Part model, mm, in its own coordinate system. Face numbers are marked on the shaded views. A direction names the side the tool comes from. Coordinates: 2 decimals unless noted, no trailing zeros. Loops run counter-clockwise (first coordinate to the right, second up) from the corner with the lowest first, then second, coordinate; pieces in that order, holes last. Notation, with made-up numbers: (60, 50) - (86, 50) arc R17 ccw to (86, 82) - close; hole circle Ø10 at (64, 21.5). An arc over 180 degrees is marked (long way). Use a Markdown table: item, result. Add a question column.
1. 3-axis set-ups, long thin cutter, end or side, ignore diameter. For the marked faces 5 and 6: which of +Z, -Z, +X, -X, +Y, -Y reach the whole face in a straight line?
2. Band-saw the part on D-D, the plane z = 20.25. Give the cut face in (x, y), plus the area to 3 significant figures.
3. Drop flat-ended pins along their axis: pin 1 (3 mm diameter, centred on x = 0, y = 0, fed in from -Z); pin 2 (2 mm diameter, centred on x = -13.5, z = 23.5, fed in from +Y); pin 3 (6 mm diameter, centred on x = 11.5, y = 11, fed in from -Z); pin 4 (5 mm diameter, centred on x = 8, y = -8.5, fed in from +Z). Give the stop position or say it passes through.
4. Pull direction Y, two halves, no side cores. Call the marked faces 1, 2, 3 and 4: pulls with the +Y half, pulls with the -Y half, needs draft (parallel to the pull), parting line crosses it, or undercut.
5. Wall check: probe 1 along X at (y, z) = (-8.5, 26.5); probe 2 along Y at (x, z) = (-8, 27.75); probe 3 along Z at (x, y) = (-8, 13). Give the ranges that are in metal, low to high. Write a range as [from, to].
6. Band-saw the part on A-A, the plane x = 0. Give the cut face in (y, z), plus the area to 3 significant figures.
7. Band-saw the part on C-C, the plane z = 24.75. Give the cut face in (x, y).
from build123d import *

# Parameters (mm, degrees)
F3_D           = 4.2
F3_CSINK_D     = 5.5
F3_CSINK_ANGLE = 90
F5_D           = 5
F5_CSINK_D     = 6.5
F5_CSINK_ANGLE = 90
F6_SIZE        = 0.3


with BuildPart() as f1:
    # F0 (on Front) → F1 (revolve)
    with BuildSketch(Plane.XZ):
        Polygon((17.5, 29.481971), (0, 29.481971), (0, 14.381971), (7.5, 14.381971), (7.5, 22.481971), (15.5, 22.481971), (15.5, 21.481971), (17.5, 21.481971), align=None)
    revolve(axis=Axis((0, 0, 21.931971), (0, 0, -1)))

    # F3 (through all)
    with Locations(Plane.XY.offset(29.481971)):
        with Locations((-8, 8.5), (8, 8.5), (8, -8.5), (-8, -8.5)):
            CounterSinkHole(F3_D / 2, F3_CSINK_D / 2, counter_sink_angle=F3_CSINK_ANGLE)

    # F5 (through all)
    with Locations(Plane(origin=(0, 0, 14.381971), x_dir=(1, 0, 0), z_dir=(0, 0, -1))):
        with Locations((0, 0)):
            CounterSinkHole(F5_D / 2, F5_CSINK_D / 2, counter_sink_angle=F5_CSINK_ANGLE)

    # F6
    f6_edges = [f1.edges().sort_by_distance(p)[0] for p in [
        (-17.5, 0, 21.481971),
    ]]
    chamfer(f6_edges, length=F6_SIZE)


solid = f1.part
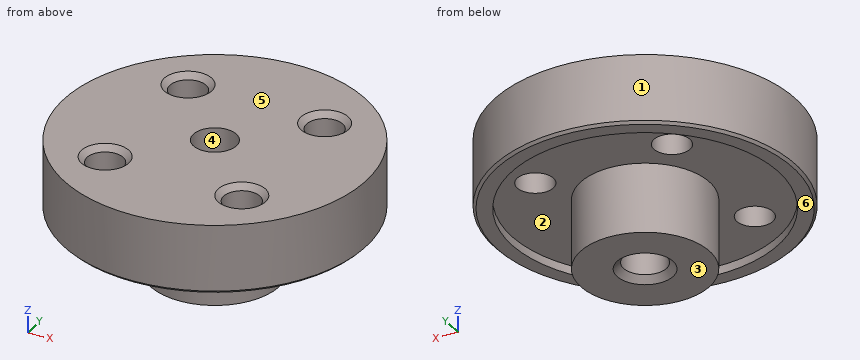
Geometry check:
| question | item | result |
|---|---|---|
| 1 | face 5 | +Z, +X, -X, +Y, -Y |
| 1 | face 6 | -Z |
| 2 | outline | circle Ø15 at (0, 0); hole circle Ø5 at (0, 0) |
| 2 | area | 157 mm^2 |
| 3 | pin 1 | passes through |
| 3 | pin 2 | stops at y = 12.25 |
| 3 | pin 3 | stops at z = 21.48 |
| 3 | pin 4 | stops at z = 29.23 |
| 4 | face 1 | parting line crosses it |
| 4 | face 2 | undercut |
| 4 | face 3 | needs draft |
| 4 | face 4 | undercut |
| 5 | probe 1 | x = [-15.3, -10.1], [-5.9, 5.9], [10.1, 15.3] |
| 5 | probe 2 | y = [-15.56, -10.6], [-6.4, 6.4], [10.6, 15.56] |
| 5 | probe 3 | z = [22.48, 29.48] |
| 6 | outline | (-17.5, 21.78) - (-17.2, 21.48) - (-15.5, 21.48) - (-15.5, 22.48) - (-7.5, 22.48) - (-7.5, 14.38) - (-3.25, 14.38) - (-2.5, 15.13) - (-2.5, 29.48) - (-17.5, 29.48) - close; (2.5, 15.13) - (3.25, 14.38) - (7.5, 14.38) - (7.5, 22.48) - (15.5, 22.48) - (15.5, 21.48) - (17.2, 21.48) - (17.5, 21.78) - (17.5, 29.48) - (2.5, 29.48) - close |
| 6 | area | 294 mm^2 |
| 7 | outline | circle Ø35 at (0, 0); hole circle Ø4.2 at (-8, -8.5); hole circle Ø4.2 at (-8, 8.5); hole circle Ø5 at (0, 0); hole circle Ø4.2 at (8, -8.5); hole circle Ø4.2 at (8, 8.5) |
